```python
from build123d import *

# Parameters (mm, degrees)
SKETCH1_W           = 6
SKETCH1_H           = 10
BOSS_EXTRUDE1_DEPTH = 8
FILLET2_RADIUS      = 3
FILLET2_LENGTH      = 10
SKETCH2_R           = 1.5
CUT_EXTRUDE1_DEPTH  = 2


with BuildPart() as part:
    # Sketch1 → Boss-Extrude1 (new body)
    with BuildSketch(Plane.XY):
        Rectangle(SKETCH1_W, SKETCH1_H)
    extrude(amount=BOSS_EXTRUDE1_DEPTH)

    # Fillet2: full round fillet: the end face becomes a half cylinder, R = half its width
    fillet2_face = Plane((0, 0, 8), x_dir=(0, -1, 0), z_dir=(0, 0, 1))  # on the end face: x along it, z out of the body
    fillet2_slab = fillet2_face.offset(-FILLET2_RADIUS / 2) * Box(FILLET2_LENGTH, 2 * FILLET2_RADIUS, FILLET2_RADIUS, mode=Mode.PRIVATE)  # the body's end, R deep
    fillet2_round = Plane((0, 0, 5), x_dir=(0, 0, 1), z_dir=(0, -1, 0)) * Cylinder(FILLET2_RADIUS, FILLET2_LENGTH, mode=Mode.PRIVATE)  # its axis R under the face
    add(fillet2_slab - fillet2_round, mode=Mode.SUBTRACT)

    # Sketch2 → Cut-Extrude1 (cut)
    with BuildSketch(Plane(origin=(0, 5, 0), x_dir=(1, 0, 0), z_dir=(0, 1, 0))):
        with Locations(Location((0, -5, 0), (0, 0, 270))):
            Circle(SKETCH2_R)
    extrude(amount=-CUT_EXTRUDE1_DEPTH, mode=Mode.SUBTRACT)


solid = part.part
```
For this review, take the finished solid that the model builds, in its own axes (mm). A direction names the side the tool comes from. Coordinates: 2 decimals unless noted, no trailing zeros. Loops run counter-clockwise (first coordinate to the right, second up) from the corner with the lowest first, then second, coordinate; pieces in that order, holes last. Notation, with made-up numbers: (7, 6.25) -> (13, 6.25) arc R9 ccw to (13, 16.25) -> close; hole circle Ø11 at (34, 22). An arc over 180 degrees is marked (long way). Return JSON: item names as keys, results as strings. Group by question number.
(1) Tool access review of faces 1 (the cylindrical face through (-0.575, 4.014, 6.386)), 2 (the flat face through (3, 0, 2)): name each direction out of +Z, -Z, +X, -X, +Y, -Y from which nothing blocks a thin tool from reaching the whole face with its end or side.
(2) For pin 1 Ø1 at (x, y) = (2, -1) entering from +Z, flat-tipped, find the tip position at first contact; note if it passes through.
(3) Mouldability with a two-part tool opening along X and no side actions: class faces 3 (the flat face through (0, 5, 3)), 4 (the cylindrical face through (0, 0, 8)), 5 (the flat face through (-3, 0, 2)), 6 (the flat face through (0, 3, 5)) as pulls with the +X half, pulls with the -X half, needs draft (parallel to the pull), parting line crosses it, or undercut.
(4) Consider section B-B, the plane z = 3.75. Give the boundary of the cut face in (x, y), plus the area to 3 significant figures.
(5) Consider section A-A, the plane x = 0. Give the boundary of the cut face in (y, z).
(6) Consider section D-D, the plane x = 2.4. Give the boundary of the cut face in (y, z).
(7) To check wall thickness, follow L1, parallel to X at y = 4.05, z = 5; L2, parallel to Y at x = -0.2, z = 6.25; L3, parallel to Z at x = -1.8, y = 2.5. State the ranges of each line that lie inside material, in increasing order.
(8) Consider section C-C, the plane y = 0.75. Give the boundary of the cut face in (x, z).
Results below:
{
 "1": {"face 1": "+Y", "face 2": "+Z, -Z, +X, +Y, -Y"},
 "2": {"pin 1": "stops at z = 7.6"},
 "3": {"face 3": "needs draft", "face 4": "parting line crosses it", "face 5": "pulls with the -X half", "face 6": "undercut"},
 "4": {"outline": "(-3, -5) -> (3, -5) -> (3, 5) -> (0.83, 5) -> (0.83, 3) -> (-0.83, 3) -> (-0.83, 5) -> (-3, 5) -> close", "area": "56.7 mm2"},
 "5": {"outline": "(-5, 0) -> (5, 0) -> (5, 3.5) -> (3, 3.5) -> (3, 6.5) -> (5, 6.5) -> (5, 8) -> (-5, 8) -> close"},
 "6": {"outline": "(-5, 0) -> (5, 0) -> (5, 6.8) -> (-5, 6.8) -> close"},
 "7": {"L1": "x = -3 to -1.5, 1.5 to 3", "L2": "y = -5 to 3", "L3": "z = 0 to 7.4"},
 "8": {"outline": "(-3, 0) -> (3, 0) -> (3, 5) arc R3 ccw to (-3, 5) -> close"}
}
